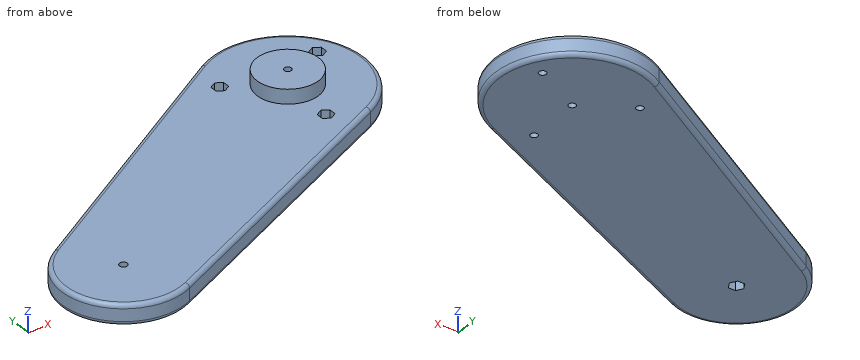
from build123d import *

# Parameters (mm, degrees)
BOSS_EXTRUDE1_DEPTH = 10
FILLET1_R           = 2
CUT_EXTRUDE8_DEPTH  = 5
CUT_EXTRUDE9_START  = -70
SKETCH10_R          = 1.75
CUT_EXTRUDE9_DEPTH  = 71
CIRPATTERN1_COUNT   = 3
SKETCH12_R          = 15
BOSS_EXTRUDE2_DEPTH = 7
CUT_EXTRUDE11_DEPTH = 5
SKETCH15_R          = 1.9
CUT_EXTRUDE12_DEPTH = 5
SKETCH16_R          = 1.75
CUT_EXTRUDE13_DEPTH = 18


with BuildPart() as part:
    # Sketch1 → Boss-Extrude1 (new body)
    with BuildSketch(Plane.XY):
        with BuildLine():
            Line((-148.531383238, -42.289811934), (-18.719283585, 32.493667415))
            ThreePointArc((-18.719283585, 32.493667415), (33.388989093, 17.071186467), (15.380384675, -34.200786062))
            Line((15.380384675, -34.200786062), (-121.25164863, -95.645374716))
            ThreePointArc((-121.25164863, -95.645374716), (-160.267147644, -81.941695039), (-148.531383238, -42.289811934))
        make_face()
    extrude(amount=BOSS_EXTRUDE1_DEPTH)

    # Fillet1
    fillet1_edges = [part.edges().sort_by_distance(p)[0] for p in [
        (33.388989093, 17.071186467, 10),
        (-83.625333411, -4.89807226, 10),
        (-160.267147644, -81.941695039, 10),
        (-83.625333411, -4.89807226, 0),
        (33.388989093, 17.071186467, 0),
        (-52.935631977, -64.923080389, 0),
        (-160.267147644, -81.941695039, 0),
        (-52.935631977, -64.923080389, 10),
    ]]
    fillet(fillet1_edges, radius=FILLET1_R)

    # Sketch3 → Cut-Extrude8 (cut)
    with BuildSketch(Plane.XY.offset(10)):
        Polygon((-4.424109202, -25.18892785), (-4.53581637, -28.767184619), (-1.492808691, -30.65305425), (1.661906157, -28.96066711), (1.773613325, -25.382410341), (-1.269394354, -23.496540711), align=None)
        Polygon((27.292728029, 14.033716876), (24.249720349, 15.919586506), (21.095005502, 14.227199366), (20.983298334, 10.648942597), (24.026306013, 8.763072967), (27.181020861, 10.455460106), align=None)
        Polygon((-19.602196811, 16.425854883), (-22.645204491, 18.311724513), (-25.799919338, 16.619337374), (-25.911626506, 13.041080604), (-22.868618827, 11.155210974), (-19.713903979, 12.847598114), align=None)
    extrude(amount=-CUT_EXTRUDE8_DEPTH, mode=Mode.SUBTRACT)

    # Sketch10 → Cut-Extrude9 (cut)
    with BuildSketch(Plane.XY.offset(5).offset(CUT_EXTRUDE9_START)):
        with Locations((24.040072147, 12.291254256)):
            Circle(SKETCH10_R)
    cut_extrude9 = extrude(amount=CUT_EXTRUDE9_DEPTH, mode=Mode.SUBTRACT)

    # CirPattern1: Cut-Extrude9 ×3 about axis
    cirpattern1_axis = Axis((0, 0, 0), (0, 0, 1))
    for i in range(1, CIRPATTERN1_COUNT):
        add(cut_extrude9.rotate(cirpattern1_axis, i * 360 / CIRPATTERN1_COUNT), mode=Mode.SUBTRACT)

    # Sketch12 → Boss-Extrude2 (add)
    with BuildSketch(Plane.XY.offset(10)):
        Circle(SKETCH12_R)
    extrude(amount=BOSS_EXTRUDE2_DEPTH)

    # Sketch14 → Cut-Extrude11 (cut)
    with BuildSketch(Plane(origin=(0, 0, 0), x_dir=(-1, 0, 0), z_dir=(0, 0, -1))):
        Polygon((137.13595637, -68.284745866), (135.34595637, -65.184374921), (131.76595637, -65.184374921), (129.97595637, -68.284745866), (131.76595637, -71.385116812), (135.34595637, -71.385116812), align=None)
    extrude(amount=-CUT_EXTRUDE11_DEPTH, mode=Mode.SUBTRACT)

    # Sketch15 → Cut-Extrude12 (cut)
    with BuildSketch(Plane(origin=(0, 0, 5), x_dir=(-1, 0, 0), z_dir=(0, 0, -1))):
        with Locations((133.55595637, -68.284745866)):
            Circle(SKETCH15_R)
    extrude(amount=-CUT_EXTRUDE12_DEPTH, mode=Mode.SUBTRACT)

    # Sketch16 → Cut-Extrude13 (cut)
    with BuildSketch(Plane(origin=(0, 0, 0), x_dir=(-1, 0, 0), z_dir=(0, 0, -1))):
        Circle(SKETCH16_R)
    extrude(amount=-CUT_EXTRUDE13_DEPTH, mode=Mode.SUBTRACT)


solid = part.part
Verification items for the finished model (mm, model axes). Coordinates: 2 decimals unless noted, no trailing zeros. Loops run counter-clockwise (first coordinate to the right, second up) from the corner with the lowest first, then second, coordinate; pieces in that order, holes last. Notation, with made-up numbers: (-24.5, -12) -> (5.5, -12) arc R31 cw to (5.5, 24) -> close; hole circle Ø7 at (77.25, 39). An arc over 180 degrees is marked (long way). Answer as a JSON object with one key per item and string values. Group by question number.
Item 1: Depth check by flat-ended pin: pin 1 (3 mm diameter, centred on x = -2, y = -27, fed in from +Z); pin 2 (3 mm diameter, centred on x = -60, y = 3, fed in from +Z); pin 3 (4.5 mm diameter, centred on x = -133.56, y = -68.28, fed in from -Z). Enter the tip coordinate at first touch or a pass-through.
Item 2: Sectioned sample at A-A on z = 14. Record the boundary of the cut face in (x, y).
Item 3: Scan lines: probe 1 along Y at (x, z) = (-1, 5.75); probe 2 along X at (y, z) = (-68.5, 6.25); probe 3 along X at (y, z) = (14, 8.5). Record each from-to range of solid material in increasing order.
Evaluation:
{
 "1": {"pin 1": "stops at z = 5", "pin 2": "stops at z = 10", "pin 3": "stops at z = 5"},
 "2": {"outline": "circle Ø30 at (0, 0); hole circle Ø3.5 at (0, 0)"},
 "3": {"probe 1": "y = -41.57 to -30.39, -23.66 to -1.44, 1.44 to 37.49", "probe 2": "x = -163.56 to -135.44, -131.67 to -60.89", "probe 3": "x = -50.69 to -25.88, -19.68 to 21.09, 27.29 to 34.72"}
}
